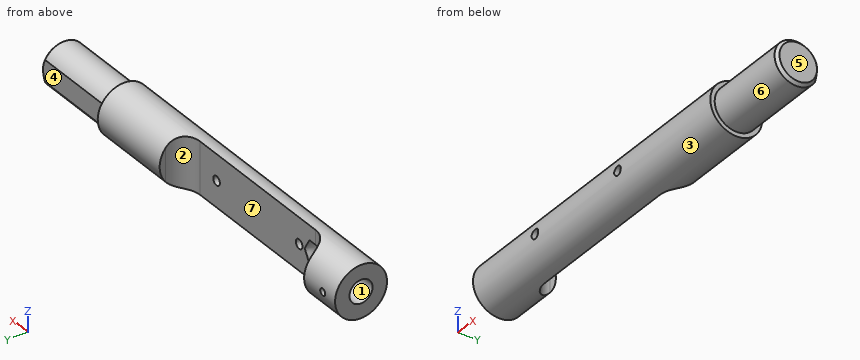
from build123d import *

# Parameters (mm, degrees)
CHANFREIN1_SIZE              = 1
ENL_V_MAT_EXTRU_1_DEPTH      = 146.557548756
ENL_V_MAT_EXTRU_1_DEPTH_BACK = 146.557548756
ESQUISSE3_W                  = 30
ESQUISSE3_H                  = 1
PER_AGE1_D                   = 8
PER_AGE1_DEPTH               = 25
PER_AGE1_TIP                 = 2.309401077
ESQUISSE6_R                  = 1.6
ENL_V_MAT_EXTRU_2_DEPTH      = 146.557548769
R_P_TITION_LIN_AIRE1_COUNT   = 2
R_P_TITION_LIN_AIRE1_PITCH   = 40
ESQUISSE7_R                  = 1.2
ENL_V_MAT_EXTRU_3_DEPTH      = 146.557548771


with BuildPart() as part:
    # Esquisse1 → Base-Révolution (revolve)
    with BuildSketch(Plane.XY, mode=Mode.PRIVATE) as base_r_volution_sk:
        Polygon((0, 0), (0, 9), (115, 9), (115, 7.5), (145, 7.5), (145, 0), align=None)
    revolve(base_r_volution_sk.sketch.rotate(Axis((0, 0, 0), (1, 0, 0)), 90), axis=Axis((0, 0, 0), (1, 0, 0)))

    # Chanfrein1
    chanfrein1_edges = [part.edges().sort_by_distance(p)[0] for p in [
        (145, 0, -7.5),
    ]]
    chamfer(chanfrein1_edges, length=CHANFREIN1_SIZE)

    # Esquisse3 → Enlèv. mat.-Extru.1 (cut, two sides: drawn at the far end of the back side and taken through both)
    with BuildSketch(Plane.XY.offset(-ENL_V_MAT_EXTRU_1_DEPTH_BACK)):
        with Locations((130, 7)):
            Rectangle(ESQUISSE3_W, ESQUISSE3_H)
        with BuildLine():
            Line((85, 9), (15, 9))
            Line((15, 9), (15, 7))
            ThreePointArc((15, 7), (17.050252532, 2.050252532), (22, 0))
            Line((22, 0), (78, 0))
            ThreePointArc((78, 0), (82.949747468, 2.050252532), (85, 7))
            Line((85, 7), (85, 9))
        make_face()
    extrude(amount=ENL_V_MAT_EXTRU_1_DEPTH + ENL_V_MAT_EXTRU_1_DEPTH_BACK, mode=Mode.SUBTRACT)

    # Perçage1
    with Locations(Plane.ZY):
        with Locations((0, 0)):
            Hole(PER_AGE1_D / 2, depth=PER_AGE1_DEPTH)
            with Locations((0, 0, -(PER_AGE1_DEPTH + PER_AGE1_TIP / 2))):  # 120° drill point
                Cone(0, PER_AGE1_D / 2, PER_AGE1_TIP, mode=Mode.SUBTRACT)

    # Esquisse6 → Enlèv. mat.-Extru.2 (cut, through all)
    with BuildSketch(Plane(origin=(0, 0, 0), x_dir=(-1, 0, 0), z_dir=(0, 1, 0))):
        with Locations(Location((-30, 0, 0), (0, 0, 90))):
            Circle(ESQUISSE6_R)
    enl_v_mat_extru_2 = extrude(amount=-ENL_V_MAT_EXTRU_2_DEPTH, mode=Mode.SUBTRACT)

    # Répétition linéaire1: Enlèv. mat.-Extru.2 ×2
    with Locations(*[(i * R_P_TITION_LIN_AIRE1_PITCH, 0, 0) for i in range(1, R_P_TITION_LIN_AIRE1_COUNT)]):
        add(enl_v_mat_extru_2, mode=Mode.SUBTRACT)

    # Esquisse7 → Enlèv. mat.-Extru.3 (cut, through all)
    with BuildSketch(Plane(origin=(0, 0, 0), x_dir=(-1, 0, 0), z_dir=(0, 1, 0))):
        with Locations(Location((-6, 0, 0), (0, 0, 270))):
            Circle(ESQUISSE7_R)
    extrude(amount=ENL_V_MAT_EXTRU_3_DEPTH, mode=Mode.SUBTRACT)


solid = part.part
Source: CAD feature listing. Evaluate the final solid. Frame: model axes, mm. Face numbers are marked on the shaded views. A direction names the side the tool comes from. Coordinates: 2 decimals unless noted, no trailing zeros. Loops run counter-clockwise (first coordinate to the right, second up) from the corner with the lowest first, then second, coordinate; pieces in that order, holes last. Notation, with made-up numbers: (-14, -6) -> (-9, -6) arc R10 cw to (-9, 13) -> close; hole circle Ø5 at (10, 14.25). An arc over 180 degrees is marked (long way). Answer in a Markdown table with one row per item. Add a question column.
Q1. Pull-direction query (X, two-part tool) for the marked faces 5, 6 and 7; classes: pulls with the +X half, pulls with the -X half, needs draft (parallel to the pull), parting line crosses it, or undercut.
Q2. Reachability of the marked faces 1, 2, 3 and 4 from +Z, -Z, +X, -X, +Y, -Y: full face, straight path, thin tool, end or side. Return the list, or none.
Q3. Section A-A on x = 70. Return the cut outline in (y, z), and give its area (3 significant figures).
Q4. Ray query, line 1 along X through (y, z) = (5.3, 0); line 2 along X through (y, z) = (5.9, 0); line 3 along Y through (x, z) = (26, -6.25). Return the intervals inside material, ascending.
Q5. Section C-C on x = 46. Return the cut outline in (y, z).
Q6. Contact query for flat-ended pins moving along their axis: pin 1 Ø1.5 at (x, y) = (105.5, 7) entering from -Z; pin 2 Ø6 at (x, z) = (130.5, 1.5) entering from +Y; pin 3 Ø4 at (x, z) = (112, -4) entering from +Y. Output: stop coordinate, or through.
Q7. Section D-D on x = 6. Return the cut outline in (y, z), and give its area (3 significant figures).
Q8. Section B-B on x = 104.5. Return the cut outline in (y, z), and give its area (3 significant figures).
Computed values:
| question | item | result |
|---|---|---|
| 1 | face 5 | pulls with the +X half |
| 1 | face 6 | needs draft |
| 1 | face 7 | undercut |
| 2 | face 1 | -X |
| 2 | face 2 | +Z, -Z, +Y |
| 2 | face 3 | +X, -X |
| 2 | face 4 | +Z, -Z, +X, +Y |
| 3 | outline | (-8.86, -1.6) arc R9 ccw to (0, -9) -> (0, -1.6) -> close; (-8.86, 1.6) -> (0, 1.6) -> (0, 9) arc R9 ccw to start |
| 3 | area | 98.6 mm^2 |
| 4 | line 1 | x = 0 to 4.8, 7.2 to 15.21, 84.79 to 145 |
| 4 | line 2 | x = 0 to 4.8, 7.2 to 15.09, 84.91 to 145 |
| 4 | line 3 | y = -6.48 to 0 |
| 5 | outline | (0, -9) -> (0, 9) arc R9 ccw to start |
| 6 | pin 1 | stops at z = -6.48 |
| 6 | pin 2 | stops at y = 6.5 |
| 6 | pin 3 | stops at y = 8.77 |
| 7 | outline | (3.82, -1.2) arc R4 cw (long way) to (3.82, 1.2) -> (8.92, 1.2) arc R9 ccw (long way) to (8.92, -1.2) -> close |
| 7 | area | 192 mm^2 |
| 8 | outline | circle Ø18 at (0, 0) |
| 8 | area | 254 mm^2 |
